from build123d import *

# Parameters (mm, degrees)
F1_DEPTH = 76.2
F2_R     = 43.31301
F2_R_2   = 18.649778
F3_DEPTH = 63.5
F4_W     = 33.762566
F4_H     = 36.540501
F5_DEPTH = 25.4


with BuildPart() as f1:
    # F0 (on Right) → F1 (new body)
    with BuildSketch(Plane.YZ):
        with BuildLine():
            ThreePointArc((-108.063558, -50.289434), (-76.870702, -33.284248), (-64.447763, 0))
            ThreePointArc((-64.447763, 0), (-76.870702, 33.284248), (-108.063558, 50.289434))
            ThreePointArc((-108.063558, 50.289434), (-166.047763, 0), (-108.063558, -50.289434))
        make_face()
        with BuildLine():
            ThreePointArc((-108.063558, 50.289434), (-76.870702, 33.284248), (-64.447763, 0))
            ThreePointArc((-64.447763, 0), (-76.870702, -33.284248), (-108.063558, -50.289434))
            Line((-108.063558, -50.289434), (67.949462, -25.144717))
            ThreePointArc((67.949462, -25.144717), (38.957359, 0), (67.949462, 25.144717))
            Line((67.949462, 25.144717), (-108.063558, 50.289434))
        make_face()
        with BuildLine():
            ThreePointArc((89.757359, 0), (83.54589, 16.642124), (67.949462, 25.144717))
            ThreePointArc((67.949462, 25.144717), (38.957359, 0), (67.949462, -25.144717))
            ThreePointArc((67.949462, -25.144717), (83.54589, -16.642124), (89.757359, 0))
        make_face()
    extrude(amount=F1_DEPTH)

    # F2 (on face) → F3 (cut)
    with BuildSketch(Plane.YZ.offset(76.2)):
        with Locations((-115.247763, 0)):
            Circle(F2_R)
        with Locations((64.357359, 0)):
            Circle(F2_R_2)
    extrude(amount=-F3_DEPTH, mode=Mode.SUBTRACT)

    # F4 (on face) → F5 (join)
    with BuildSketch(Plane.YZ.offset(76.2)):
        with Locations((-21.275819, -2.24594)):
            Rectangle(F4_W, F4_H)
    extrude(amount=F5_DEPTH)


solid = f1.part
Input: part model. Units: mm. Frame: model coordinates. A direction names the side the tool comes from. Coordinates: 2 decimals unless noted, no trailing zeros. Order: outer loops, then holes, each group sorted by start corner. A loop starts at its lowest first (then second) coordinate and runs counter-clockwise, first axis right, second up. Notation, with made-up numbers: M 20,86.5 L 41,86.5 A21 cw 41,93.5 Z; hole C 8,-21.5 d1. An arc over 180 degrees is marked long. One line per question, with ' | ' between items.
Item 1: Ray query, line 1 along Y through (x, z) = (70, -4); line 2 along Z through (x, y) = (97, -17); line 3 along X through (y, z) = (10.5, 20.5). Return the intervals inside material, ascending.
Geometry results:
line 1: y = -165.89 to -158.38, -72.12 to 46.14, 82.57 to 89.44 | line 2: z = -20.52 to 16.02 | line 3: x = 0 to 76.2
Item 2: Section C-C (z = 9). Output: boundary loops of the cut face in (x, y), then the cut area to 3 significant figures.
Geometry results:
outline: M 0,-165.24 L 76.2,-165.24 L 76.2,-157.62 L 12.7,-157.62 L 12.7,-72.88 L 76.2,-72.88 L 76.2,-38.16 L 101.6,-38.16 L 101.6,-4.39 L 76.2,-4.39 L 76.2,48.02 L 12.7,48.02 L 12.7,80.69 L 76.2,80.69 L 76.2,88.11 L 0,88.11 Z | area: 12,700 mm^2
Item 3: Section B-B (y = -79). Output: boundary loops of the cut face in (x, z), then the cut area to 3 significant figures.
Geometry results:
outline: M 0,-46.14 L 76.2,-46.14 L 76.2,-23.71 L 12.7,-23.71 L 12.7,23.71 L 76.2,23.71 L 76.2,46.14 L 0,46.14 Z | area: 4,020 mm^2
Item 4: Draft query along Z for faces 5 (the cylindrical face through (44.89, -75.24, -16.59)), 6 (the flat face through (89, -22, 16.024)), 7 (the flat face through (12.7, 64, 0)), 8 (the flat face through (76.2, -40, 1)). Return one class per face: released by +Z, released by -Z, zero draft, split by the parting line, or undercut.
Geometry results:
face 5: undercut | face 6: released by +Z | face 7: undercut | face 8: zero draft
Item 5: Section D-D (x = 81.5). Output: boundary loops of the cut face in (y, z), then the cut area to 3 significant figures.
Geometry results:
outline: M -38.16,-20.52 L -4.39,-20.52 L -4.39,16.02 L -38.16,16.02 Z | area: 1,230 mm^2
Item 6: Reachability of faces 1 (the flat face through (89, -22, -20.516)), 2 (the cylindrical face through (44.894, 45.726, 0.82)), 3 (the flat face through (89, -4.395, -3)), 4 (the flat face through (89, -38.157, -3)) from +Z, -Z, +X, -X, +Y, -Y: full face, straight path, thin tool, end or side. Return the list, or none.
Geometry results:
face 1: -Z, +X, +Y, -Y | face 2: +X | face 3: +Z, -Z, +X, +Y | face 4: +Z, -Z, +X, -Y
Item 7: Section A-A (x = 31). Output: boundary loops of the cut face in (y, z), then the cut area to 3 significant figures.
Geometry results:
outline: M -108.06,-50.29 L 67.95,-25.14 A25.4 ccw 89.76,0 A25.4 ccw 67.95,25.14 L -108.06,50.29 A50.8 ccw long Z; hole C -115.25,0 d86.63; hole C 64.36,0 d37.3 | area: 11,900 mm^2
Item 8: Pin query (flat end, axial travel): pin 1 (12.5 mm diameter, centred on x = 83.5, z = -5, fed in from +Y); pin 2 (7.5 mm diameter, centred on x = 94.5, y = -20.5, fed in from +Z); pin 3 (2 mm diameter, centred on x = 67, y = -93, fed in from -Z). Return the tip coordinate at first contact, or that it passes through.
Geometry results:
pin 1: stops at y = -4.39 | pin 2: stops at z = 16.02 | pin 3: stops at z = -48.28
